Verification items for the finished model (mm, model axes). Face numbers are marked on the shaded views. Give positions to 0.01 mm unless a question says otherwise; leave off trailing zeros. Order: outer loops, then holes, each group sorted by start corner. A loop starts at its lowest first (then second) coordinate and runs counter-clockwise, first axis right, second up. Notation, with made-up numbers: (-28, 25) - (-4, 25) arc R24 ccw to (-4, 63) - close; hole circle Ø6 at (19, -18). An arc over 180 degrees is marked (long way). Answer as a JSON object with one key per item and string values.
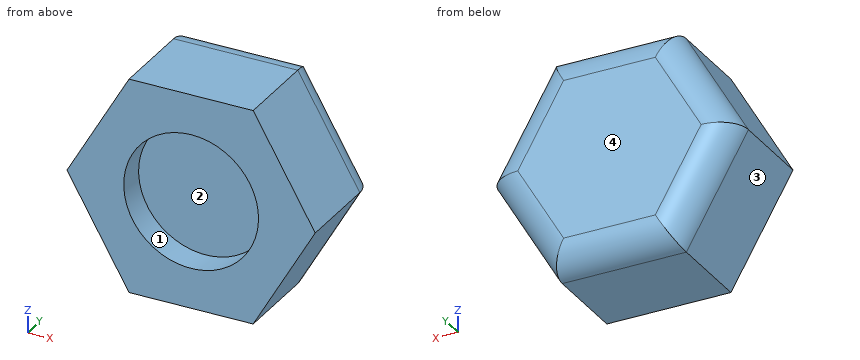
```python
from build123d import *

# Parameters (mm, degrees)
SKETCH1_R           = 2.4
BOSS_EXTRUDE1_DEPTH = 4
FILLET1_R           = 1
BOSS_EXTRUDE4_START = -3
SKETCH2_R           = 2.4
BOSS_EXTRUDE4_DEPTH = 3


with BuildPart() as part:
    # Sketch1 → Boss-Extrude1 (new body)
    with BuildSketch(Plane(origin=(0, 0, 0), x_dir=(1, 0, 0), z_dir=(0, 1, 0))):
        Polygon((-4.419962439, 0), (-2.20998122, -3.827799756), (2.20998122, -3.827799756), (4.419962439, 0), (2.20998122, 3.827799756), (-2.20998122, 3.827799756), align=None)
        with Locations(Location((0, 0, 0), (0, 0, 270))):
            Circle(SKETCH1_R, mode=Mode.SUBTRACT)
    extrude(amount=BOSS_EXTRUDE1_DEPTH)

    # Fillet1
    fillet1_edges = [part.edges().sort_by_distance(p)[0] for p in [
        (0, 4, 3.827799756),
        (3.31497183, 4, 1.913899878),
        (3.31497183, 4, -1.913899878),
        (0, 4, -3.827799756),
        (-3.31497183, 4, -1.913899878),
        (-3.31497183, 4, 1.913899878),
    ]]
    fillet(fillet1_edges, radius=FILLET1_R)

    # Sketch2 → Boss-Extrude4 (add)
    with BuildSketch(Plane(origin=(0, 4, 0), x_dir=(1, 0, 0), z_dir=(0, 1, 0)).offset(BOSS_EXTRUDE4_START)):
        with Locations(Location((0, 0, 0), (0, 0, 270))):
            Circle(SKETCH2_R)
    extrude(amount=BOSS_EXTRUDE4_DEPTH)


solid = part.part
```
(1) Section check D-D (x = 1.25). Record the cut outline in (y, z), then the cut area to 3 significant figures.
Computed values:
{"outline": "(0, -3.83) - (3, -3.83) arc R1 ccw to (4, -2.83) - (4, 2.83) arc R1 ccw to (3, 3.83) - (0, 3.83) - (0, 2.05) - (1, 2.05) - (1, -2.05) - (0, -2.05) - close", "area": "26.1 mm²"}
(2) Gauge pin test, flat end, axial feed: pin 1 Ø2 at (y, z) = (1.5, -2.5) entering from -X. Record the tip position at first contact, or that the pin passes through.
Computed values:
{"pin 1": "stops at x = -3.55"}
(3) Material ranges on line 1 along Y through (x, z) = (0.75, -1); line 2 along X through (y, z) = (2.95, 2); line 3 along X through (y, z) = (0.85, -0.25), recorded low to high. Write a range as [from, to].
Computed values:
{"line 1": "y = [1, 4]", "line 2": "x = [-3.27, 3.27]", "line 3": "x = [-4.28, -2.39], [2.39, 4.28]"}
(4) Section check B-B (x = 0). Record the cut outline in (y, z), then the cut area to 3 significant figures.
Computed values:
{"outline": "(0, -3.83) - (3, -3.83) arc R1 ccw to (4, -2.83) - (4, 2.83) arc R1 ccw to (3, 3.83) - (0, 3.83) - (0, 2.4) - (1, 2.4) - (1, -2.4) - (0, -2.4) - close", "area": "25.4 mm²"}
(5) Section check C-C (y = 3.2). Record the cut outline in (x, z).
Computed values:
{"outline": "(-4.4, 0) - (-2.2, -3.81) - (2.2, -3.81) - (4.4, 0) - (2.2, 3.81) - (-2.2, 3.81) - close"}
(6) Section check A-A (y = 0.85). Record the cut outline in (x, z).
Computed values:
{"outline": "(-4.42, 0) - (-2.21, -3.83) - (2.21, -3.83) - (4.42, 0) - (2.21, 3.83) - (-2.21, 3.83) - close; hole circle Ø4.8 at (0, 0)"}
(7) Release check for a two-part mould opening along X. For the marked faces 1, 2, 3 and 4 record: pulls with the +X half, pulls with the -X half, needs draft (parallel to the pull), parting line crosses it, or undercut.
Computed values:
{"face 1": "undercut", "face 2": "undercut", "face 3": "pulls with the -X half", "face 4": "needs draft"}
